Part print with two shaded views. Sizes in mm from the minimum x, y, z corner. A direction names the side the tool comes from. Round coordinates to 2 decimals unless told otherwise and drop trailing zeros. Order: outer loops, then holes, each group sorted by start corner. A loop starts at its lowest first (then second) coordinate and runs counter-clockwise, first axis right, second up. Notation, with made-up numbers: M 80,29 L 102,29 A24 cw 102,53 Z; hole C 2,70.5 d3. An arc over 180 degrees is marked long. One line per question, with ' | ' between items.
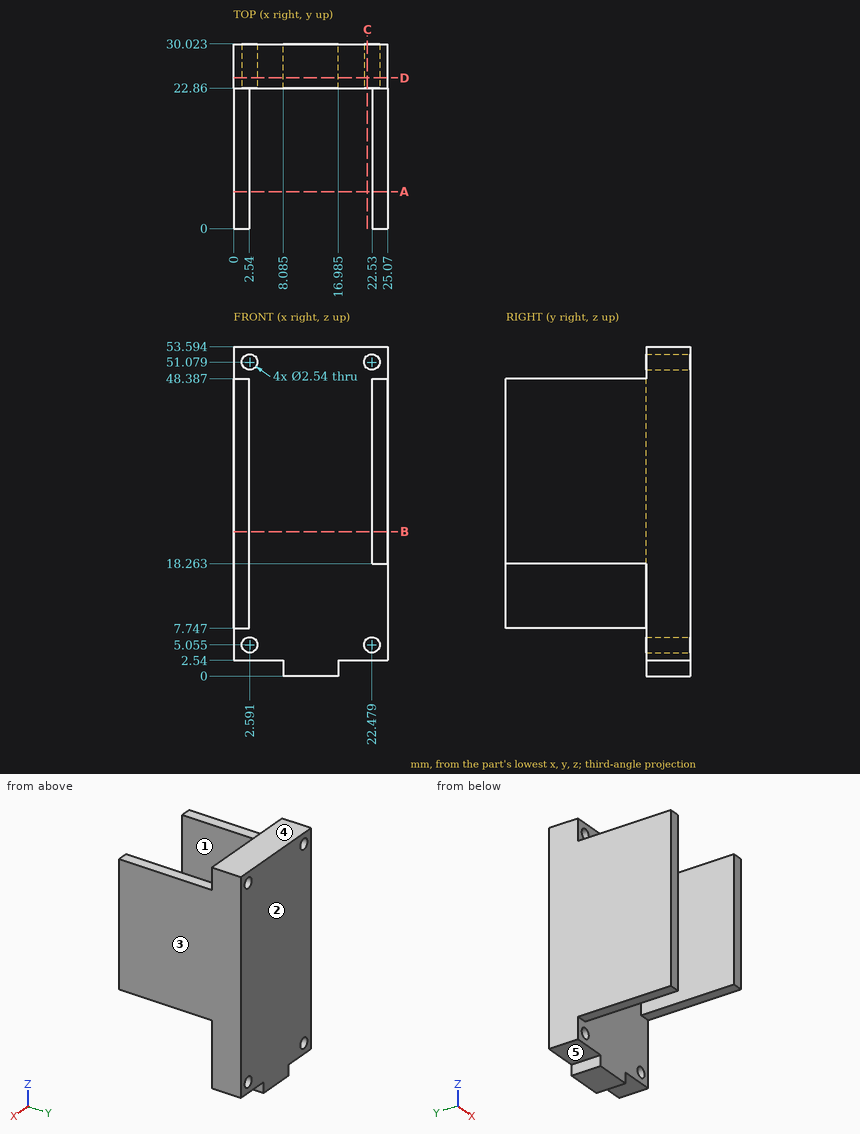
1) Saw through at C-C (x = 21.75). List the corners of the cut face in (y, z) (1 decimal).
The answers:
outline: M 22.9,2.5 L 30,2.5 L 30,4 L 22.9,4 Z; M 22.9,6.1 L 30,6.1 L 30,50 L 22.9,50 Z; M 22.9,52.1 L 30,52.1 L 30,53.6 L 22.9,53.6 Z
2) Which spindle directions (+Z, -Z, +X, -X, +Y, -Y) get a long thin tool onto all of the face, cutting with end or side? Do the marked faces 1 and 2. Say none if no direction does.
The answers:
face 1: +Z, -Z, -Y | face 2: +Z, -Z, +X, -X, +Y
3) Probe line 1 (X direction, y = 10, z = 22); line 2 (Z direction, x = 1.75, y = 25) (1 decimal); line 3 (Y direction, x = 8.25, z = 11.5). List the from-to ranges inside material, lowest first. Write a range as [from, to].
The answers:
line 1: x = [0, 2.54], [22.53, 25.07] | line 2: z = [2.5, 4.1], [6, 50.1], [52, 53.6] | line 3: y = [22.86, 30.02]
4) Saw through at D-D (y = 24.5). Give the number of separate pieces and of enclosed holes in the cut face, plus the area to 3 significant figures.
The answers:
separate pieces: 1 | enclosed holes: 4 | area: 1,280 mm²
5) Drop flat-ended pins along their axis: pin 1 (6 mm diameter, centred on x = 3.5, y = 27, fed in from -Z); pin 2 (3 mm diameter, centred on x = 1, y = 14.5, fed in from +Z); pin 3 (3 mm diameter, centred on x = 1, y = 13.5, fed in from -Z); pin 4 (2 mm diameter, centred on x = 22.48, z = 51.08, fed in from +Y). Give the stop position or say it passes through.
The answers:
pin 1: stops at z = 2.54 | pin 2: stops at z = 48.39 | pin 3: stops at z = 7.75 | pin 4: passes through
6) Saw through at A-A (y = 6). List the corners of the cut face in (x, z).
The answers:
outline: M 0,7.75 L 2.54,7.75 L 2.54,48.39 L 0,48.39 Z; M 22.53,18.26 L 25.07,18.26 L 25.07,48.39 L 22.53,48.39 Z
7) Two-plate mould, pull along Z, no slides. Class the marked faces 3, 4 and 5: released by +Z, released by -Z, zero draft, split by the parting line, or undercut.
The answers:
face 3: zero draft | face 4: released by +Z | face 5: released by -Z
8) Saw through at B-B (z = 23.5). List the corners of the cut face in (x, y), plus the area to 3 significant figures.
The answers:
outline: M 0,0 L 2.54,0 L 2.54,22.86 L 22.53,22.86 L 22.53,0 L 25.07,0 L 25.07,30.02 L 0,30.02 Z | area: 296 mm²
